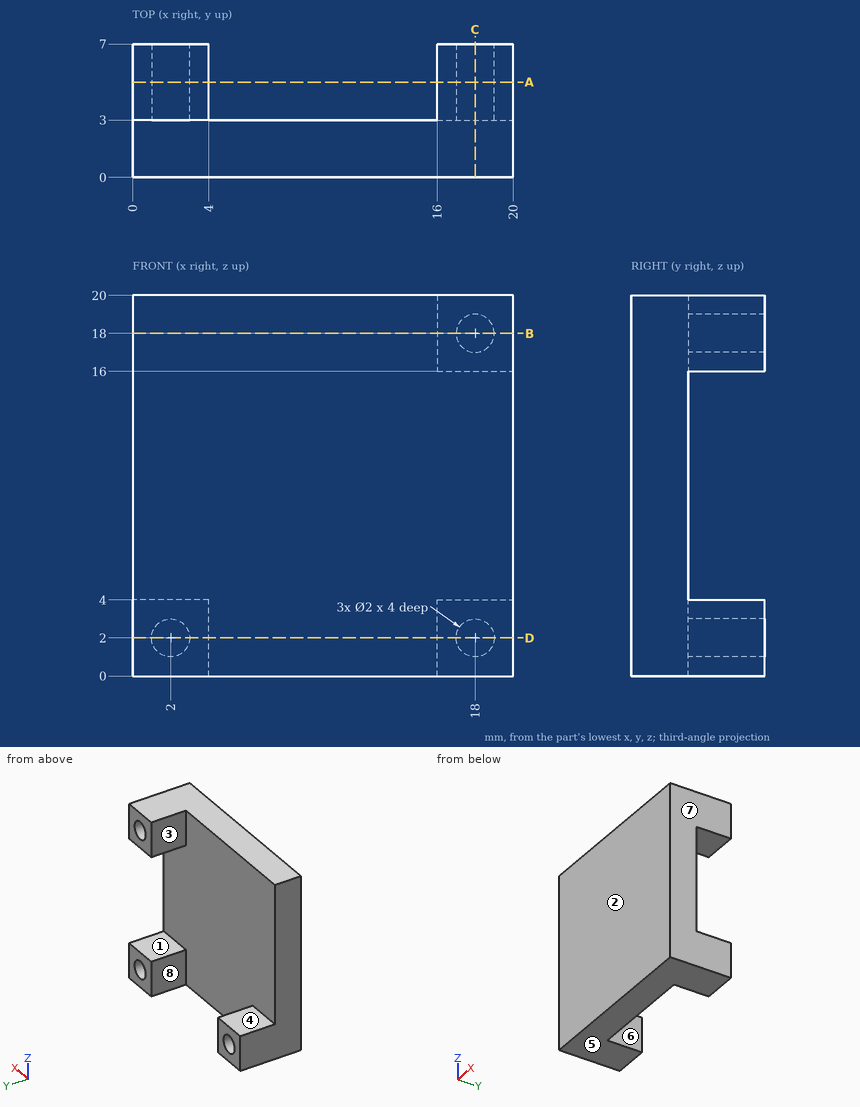
The figure shows three views and two pictorial views of one solid part (mm, origin at its lowest corner). Answer the questions. A direction names the side the tool comes from. Give positions to 0.01 mm unless a question says otherwise; leave off trailing zeros. Write each loop counter-clockwise with the first axis right and the second up, starting at its lowest first coordinate (ties: lowest second). Pieces come first, ordered by that corner, then holes. Notation, with made-up numbers: (57, 13.5) -> (106, 13.5) arc R18 cw to (106, 33.5) -> close; hole circle Ø6 at (83.5, 48.5). An arc over 180 degrees is marked (long way). Answer as a JSON object with one key per item and string values.
1) Section C-C on x = 18 is taken. Write down the section's boundary in (y, z), then the cut area to 3 significant figures.
Findings below:
{"outline": "(0, 0) -> (7, 0) -> (7, 1) -> (3, 1) -> (3, 3) -> (7, 3) -> (7, 4) -> (3, 4) -> (3, 16) -> (7, 16) -> (7, 17) -> (3, 17) -> (3, 19) -> (7, 19) -> (7, 20) -> (0, 20) -> close", "area": "76.0 mm^2"}
2) A tool of negligible diameter and unlimited length cuts with its end or side. For the marked faces 1, 2, 3 and 4, from which of +Z, -Z, +X, -X, +Y, -Y can it reach the whole face along a straight path? Write none if from no direction.
Findings below:
{"face 1": "+X, -X, +Y", "face 2": "+Z, -Z, +X, -X, -Y", "face 3": "+Z, -Z, -X, +Y", "face 4": "+Z, +X, -X, +Y"}
3) Flat-ended cylindrical pins translate along their axes: pin 1 Ø1.6 at (x, z) = (2, 2) entering from +Y; pin 2 Ø1.2 at (y, z) = (5, 18.5) entering from -X; pin 3 Ø3 at (x, y) = (2.5, 5.5) entering from +Z. Find the tip coordinate at first contact, or state that the pin passes through.
Findings below:
{"pin 1": "stops at y = 3", "pin 2": "stops at x = 16", "pin 3": "stops at z = 4"}
4) Section B-B on z = 18 is taken. Write down the section's boundary in (x, y), then the cut area to 3 significant figures.
Findings below:
{"outline": "(0, 0) -> (20, 0) -> (20, 7) -> (19, 7) -> (19, 3) -> (17, 3) -> (17, 7) -> (16, 7) -> (16, 3) -> (0, 3) -> close", "area": "68.0 mm^2"}
5) Straight lines are drawn through the part: probe 1 along X at (y, z) = (5.1, 2); probe 2 along Z at (x, y) = (2, 4.75). For each, find the intervals that lie inside material, in ascending order. Write a range as from..to.
Findings below:
{"probe 1": "x = 0..1, 3..4, 16..17, 19..20", "probe 2": "z = 0..1, 3..4"}
6) Section D-D on z = 2 is taken. Write down the section's boundary in (x, y).
Findings below:
{"outline": "(0, 0) -> (20, 0) -> (20, 7) -> (19, 7) -> (19, 3) -> (17, 3) -> (17, 7) -> (16, 7) -> (16, 3) -> (4, 3) -> (4, 7) -> (3, 7) -> (3, 3) -> (1, 3) -> (1, 7) -> (0, 7) -> close"}
7) Section A-A on y = 5 is taken. Write down the section's boundary in (x, z), then the cut area to 3 significant figures.
Findings below:
{"outline": "(0, 0) -> (4, 0) -> (4, 4) -> (0, 4) -> close; (16, 0) -> (20, 0) -> (20, 4) -> (16, 4) -> close; (16, 16) -> (20, 16) -> (20, 20) -> (16, 20) -> close; hole circle Ø2 at (2, 2); hole circle Ø2 at (18, 2); hole circle Ø2 at (18, 18)", "area": "38.6 mm^2"}
8) For a pull along X with two mould halves and no side action, classify the marked faces 5, 6, 7 and 8 as pulls with the +X half, pulls with the -X half, needs draft (parallel to the pull), parting line crosses it, or undercut.
Findings below:
{"face 5": "needs draft", "face 6": "undercut", "face 7": "pulls with the +X half", "face 8": "undercut"}
